from build123d import *

# Parameters (mm, degrees)
F0_W     = 60
F0_H     = 12.951542
F0_R     = 0.709255
F0_R_2   = 1.95
F0_R_3   = 2
F0_R_4   = 2.05
F0_R_5   = 2.1
F0_R_6   = 2.15
F1_DEPTH = 8
F2_DEPTH = 5
F3_SIZE  = 0.5


with BuildPart() as f1:
    # F0 (on Top) → F1 (new body)
    with BuildSketch(Plane.XY):
        Rectangle(F0_W, F0_H)
        with Locations((-28.05865, -4.393477)):
            Circle(F0_R, mode=Mode.SUBTRACT)
        with Locations((-24, 0)):
            Circle(F0_R_2, mode=Mode.SUBTRACT)
        with Locations((-12, 0)):
            Circle(F0_R_3, mode=Mode.SUBTRACT)
        Circle(F0_R_4, mode=Mode.SUBTRACT)
        with Locations((12, 0)):
            Circle(F0_R_5, mode=Mode.SUBTRACT)
        with Locations((24, 0)):
            Circle(F0_R_6, mode=Mode.SUBTRACT)
    extrude(amount=F1_DEPTH)

    # F0 (on Top) → F2 (join)
    with BuildSketch(Plane.XY):
        with Locations((-28.05865, -4.393477)):
            Circle(F0_R)
    extrude(amount=F2_DEPTH)

    # F3
    f3_edges = [f1.edges().sort_by_distance(p)[0] for p in [
        (-25.95, 0, 8),
        (-14, 0, 8),
        (-2.05, 0, 8),
        (9.9, 0, 8),
        (21.85, 0, 8),
        (21.85, 0, 0),
        (9.9, 0, 0),
        (-2.05, 0, 0),
        (-14, 0, 0),
        (-25.95, 0, 0),
        (-30, -6.475771, 4),
        (-30, 6.475771, 4),
        (30, 6.475771, 4),
        (30, -6.475771, 4),
    ]]
    chamfer(f3_edges, length=F3_SIZE)


solid = f1.part
Build history of the part. All positions in model axes, mm. Round coordinates to 2 decimals unless told otherwise and drop trailing zeros. Order: outer loops, then holes, each group sorted by start corner. A loop starts at its lowest first (then second) coordinate and runs counter-clockwise, first axis right, second up. Notation, with made-up numbers: M 60,19 L 64,19 A20 ccw 64,49 Z; hole C 71.5,55.25 d1. An arc over 180 degrees is marked long. Use CSV: the item, a comma, the result in double quotes. Start each with the question number.
(1) Drill centre lines: probe 1 along X at (y, z) = (-0.5, 4); probe 2 along X at (y, z) = (-1.5, 3.5); probe 3 along Y at (x, z) = (-23, 2.75). Where is each one in solid material? Low to high.
(2) Cut at B-B on z = 4. List the corners of the cut face in (x, y).
(3) Flat gauge pins, fed straight in: P1, Ø1.3, axis at x = -28.06, y = -4.39, coming from the +Z side; P2, Ø4.5, axis at x = -24, y = 0, coming from the -Z side. Where does each tip first touch, or does it go through?
(4) Cut at D-D on y = 0. State how many separate pieces and enclosed holes the cut face has, then the cut area to 4 significant figures.
(5) Cut at A-A on x = -12. List the corners of the cut face in (y, z), then the cut area to 3 significant figures.
(6) Mould opens along X. For faces 1 (the face through (-27.403, -4.665, 6.479)), 2 (the face through (0, 6.476, 4)), 3 (the face through (-30, 0, 4)) say: +X half, -X half, draft (parallel to the pull), parting line (faces both ways), or undercut.
(7) Cut at C-C on x = 12. List the corners of the cut face in (y, z).
Findings:
1,probe 1,"x = -30 to -25.88, -22.12 to -13.94, -10.06 to -1.99, 1.99 to 9.96, 14.04 to 21.91, 26.09 to 30"
1,probe 2,"x = -30 to -25.25, -22.75 to -13.32, -10.68 to -1.4, 1.4 to 10.53, 13.47 to 22.46, 25.54 to 30"
1,probe 3,"y = -6.48 to -1.67, 1.67 to 6.48"
2,outline,"M -30,-5.98 L -29.5,-6.48 L 29.5,-6.48 L 30,-5.98 L 30,5.98 L 29.5,6.48 L -29.5,6.48 L -30,5.98 Z; hole C -24,0 d3.9; hole C -12,0 d4; hole C 0,0 d4.1; hole C 12,0 d4.2; hole C 24,0 d4.3"
3,P1,"stops at z = 5"
3,P2,"stops at z = 0.2"
4,separate pieces,"6"
4,enclosed holes,"0"
4,area,"313.5 mm^2"
5,outline,"M -6.48,0 L -2.5,0 L -2,0.5 L -2,7.5 L -2.5,8 L -6.48,8 Z; M 2,0.5 L 2.5,0 L 6.48,0 L 6.48,8 L 2.5,8 L 2,7.5 Z"
5,area,"71.1 mm^2"
6,face 1,"undercut"
6,face 2,"draft"
6,face 3,"-X half"
7,outline,"M -6.48,0 L -2.6,0 L -2.1,0.5 L -2.1,7.5 L -2.6,8 L -6.48,8 Z; M 2.1,0.5 L 2.6,0 L 6.48,0 L 6.48,8 L 2.6,8 L 2.1,7.5 Z"
